Geometry check sheet. Reference: the model listing, model coordinates, mm. Round coordinates to 2 decimals unless told otherwise and drop trailing zeros. Loops run counter-clockwise (first coordinate to the right, second up) from the corner with the lowest first, then second, coordinate; pieces in that order, holes last. Notation, with made-up numbers: (82.25, 76.5) - (128.25, 76.5) arc R16 cw to (128.25, 82.5) - close; hole circle Ø1 at (18.5, 22). An arc over 180 degrees is marked (long way). Answer in a Markdown table with one row per item. Add a question column.
```python
from build123d import *

# Parameters (mm, degrees)
SKETCH1_W                   = 1090.6125
SKETCH1_H                   = 298.45
BOSS_EXTRUDE1_DEPTH         = 3.175
SKETCH2_W                   = 9.525
SKETCH2_H                   = 203.2
CUT_EXTRUDE1_DEPTH          = 4.175
FILLET1_R                   = 3.175
FILLET1_OF_MIRROR1_R        = 3.175
F_1_4_0_25_DIAMETER_HOLE1_D = 6.35
FILLET2_R                   = 3.175


with BuildPart() as part:
    # Sketch1 → Boss-Extrude1 (new body)
    with BuildSketch(Plane(origin=(0, 0, 0), x_dir=(1, 0, 0), z_dir=(0, 1, 0))):
        Rectangle(SKETCH1_W, SKETCH1_H)
    extrude(amount=BOSS_EXTRUDE1_DEPTH)

    # Sketch2 → Cut-Extrude1 (cut, through all)
    with BuildSketch(Plane(origin=(0, 3.175, 0), x_dir=(1, 0, 0), z_dir=(0, 1, 0))):
        with Locations((540.54375, 0)):
            Rectangle(SKETCH2_W, SKETCH2_H)
    cut_extrude1 = extrude(amount=-CUT_EXTRUDE1_DEPTH, mode=Mode.SUBTRACT)

    # Fillet1
    fillet1_edges = [part.edges().sort_by_distance(p)[0] for p in [
        (535.78125, 1.5875, 101.6),
        (535.78125, 1.5875, -101.6),
    ]]
    fillet(fillet1_edges, radius=FILLET1_R)

    # Mirror1: Cut-Extrude1 across plane
    add(cut_extrude1.mirror(Plane(origin=(0, 0, 0), x_dir=(0, 0, 1), z_dir=(1, 0, 0))), mode=Mode.SUBTRACT)

    # Fillet1 of Mirror1
    fillet1_of_mirror1_edges = [part.edges().sort_by_distance(p)[0] for p in [
        (-535.78125, 1.5875, 101.6),
        (-535.78125, 1.5875, -101.6),
    ]]
    fillet(fillet1_of_mirror1_edges, radius=FILLET1_OF_MIRROR1_R)

    # 1/4 (0.25) Diameter Hole1 (through all)
    with Locations(Plane(origin=(0, 3.175, 0), x_dir=(1, 0, 0), z_dir=(0, 1, 0))):
        with Locations((482.6, 142.875), (0, 142.875), (-482.6, 142.875)):
            f_1_4_0_25_diameter_hole1 = Hole(F_1_4_0_25_DIAMETER_HOLE1_D / 2)

    # Mirror2: 1/4 (0.25) Diameter Hole1 across plane
    add(f_1_4_0_25_diameter_hole1.mirror(Plane.XY), mode=Mode.SUBTRACT)

    # Fillet2
    fillet2_edges = [part.edges().sort_by_distance(p)[0] for p in [
        (545.30625, 1.5875, -101.6),
        (545.30625, 1.5875, 101.6),
        (-545.30625, 1.5875, 101.6),
        (-545.30625, 1.5875, -101.6),
        (545.30625, 1.5875, 149.225),
        (-545.30625, 1.5875, 149.225),
        (-545.30625, 1.5875, -149.225),
        (545.30625, 1.5875, -149.225),
    ]]
    fillet(fillet2_edges, radius=FILLET2_R)


solid = part.part
```
Q1. Scan lines: line 1 (Z direction, x = 0, y = 0.8) (3 decimals); line 2 (X direction, y = 2.85, z = 1.5). Record each from-to range of solid material in increasing order. Write a range as from..to.
Q2. Cross-section at A-A, the plane z = -85.5. Enter the section's corners in (x, y) (3 decimals).
Q3. Depth check by flat-ended pin: P1, Ø5, axis at x = -482.6, z = 142.875, coming from the +Y side; P2, Ø1.6, axis at y = 2, z = 22, coming from the -X side. Enter the tip coordinate at first touch or a pass-through.
Check sheet entries:
| question | item | result |
|---|---|---|
| 1 | line 1 | -149.225..-146.05, -139.7..139.7, 146.05..149.225 |
| 1 | line 2 | -535.78..535.78 |
| 2 | outline | (-535.781, 0) - (535.781, 0) - (535.781, 3.175) - (-535.781, 3.175) - close |
| 3 | P1 | through |
| 3 | P2 | x = -535.78 |
